Here's how the part is built. I have some questions about the finished solid (model axes, mm). Face numbers are marked on the shaded views. A direction names the side the tool comes from. Coordinates: 2 decimals unless noted, no trailing zeros. Write each loop counter-clockwise with the first axis right and the second up, starting at its lowest first coordinate (ties: lowest second). Pieces come first, ordered by that corner, then holes.
Item 1: If I drill on line 1 (X direction, y = -5, z = 4.5); line 2 (X direction, y = -3.75, z = 4); line 3 (X direction, y = -25.5, z = 5.5), over which ranges is the centre line in solid material (lowest first)?
Item 2: If we section it at B-B (z = -21.5): Please give me the cut outline in (x, y) (3 decimals).
Item 3: We'd pull the mould along Z, two halves only. Please class the marked faces 1, 2 and 3: +Z half, -Z half, draft (parallel to the pull), parting line (faces both ways), or undercut.
Item 4: If we section it at A-A (y = -13): Please give me the cut outline in (x, z), then the cut area to 3 significant figures.
Item 5: If we section it at D-D (y = -23): Please give me the cut outline in (x, z), then the cut area to 3 significant figures.
Item 6: For the marked faces 4, 5 and 6, which set-ups out of +Z, -Z, +X, -X, +Y, -Y let a thin tool reach every point of the face, with its end or its side?
Item 7: I'm going to push flat-ended pins straight in: pin 1 Ø18 at (x, z) = (-15, 0) entering from -Y; pin 2 Ø6 at (x, y) = (-22.5, -24) entering from -Z; pin 3 Ø3 at (x, y) = (-25, -8.5) entering from -Z. Where does each tip first touch, or does it pass through?
Item 8: If we section it at C-C (x = -16): Please give me the cut outline in (y, z), then the cut area to 3 significant figures.
from build123d import *

# Parameters (mm, degrees)
F1_DEPTH = 1
F2_DEPTH = 20
F3_DEPTH = 27


with BuildPart() as f1:
    # F0 (on Front) → F1 (new body)
    with BuildSketch(Plane.XZ):
        with BuildLine():
            ThreePointArc((28.6, -10.2), (24.1268833673, 14.3422452914), (0, 8))
            ThreePointArc((0, 8), (-24.1268833673, 14.3422452914), (-28.6, -10.2))
            Line((-28.6, -10.2), (0, -48.3333333333))
            Line((0, -48.3333333333), (28.6, -10.2))
        make_face()
        with BuildLine():
            ThreePointArc((-27.64, -9.48), (-22.3177005427, 14.0032588624), (0, 4.9638694584))
            ThreePointArc((0, 4.9638694584), (22.3177005427, 14.0032588624), (27.64, -9.48))
            Line((27.64, -9.48), (0, -46.3333333333))
            Line((0, -46.3333333333), (-27.64, -9.48))
        make_face(mode=Mode.SUBTRACT)
        with BuildLine():
            ThreePointArc((27.64, -9.48), (22.3177005427, 14.0032588624), (0, 4.9638694584))
            ThreePointArc((0, 4.9638694584), (-22.3177005427, 14.0032588624), (-27.64, -9.48))
            Line((-27.64, -9.48), (0, -46.3333333333))
            Line((0, -46.3333333333), (27.64, -9.48))
        make_face()
        with BuildLine():
            ThreePointArc((-27, -9), (-19.7434164903, 14.2302494708), (0, 0))
            ThreePointArc((0, 0), (19.7434164903, 14.2302494708), (27, -9))
            Line((27, -9), (0, -45))
            Line((0, -45), (-27, -9))
        make_face(mode=Mode.SUBTRACT)
        with BuildLine():
            ThreePointArc((27, -9), (19.7434164903, 14.2302494708), (0, 0))
            ThreePointArc((0, 0), (-19.7434164903, 14.2302494708), (-27, -9))
            Line((-27, -9), (0, -45))
            Line((0, -45), (27, -9))
        make_face()
    extrude(amount=F1_DEPTH)

    # F0 (on Front) → F2 (join)
    with BuildSketch(Plane.XZ):
        with BuildLine():
            ThreePointArc((28.6, -10.2), (24.1268833673, 14.3422452914), (0, 8))
            ThreePointArc((0, 8), (-24.1268833673, 14.3422452914), (-28.6, -10.2))
            Line((-28.6, -10.2), (0, -48.3333333333))
            Line((0, -48.3333333333), (28.6, -10.2))
        make_face()
        with BuildLine():
            ThreePointArc((-27.64, -9.48), (-22.3177005427, 14.0032588624), (0, 4.9638694584))
            ThreePointArc((0, 4.9638694584), (22.3177005427, 14.0032588624), (27.64, -9.48))
            Line((27.64, -9.48), (0, -46.3333333333))
            Line((0, -46.3333333333), (-27.64, -9.48))
        make_face(mode=Mode.SUBTRACT)
    extrude(amount=F2_DEPTH)

    # F0 (on Front) → F3 (join)
    with BuildSketch(Plane.XZ):
        with BuildLine():
            ThreePointArc((27.64, -9.48), (22.3177005427, 14.0032588624), (0, 4.9638694584))
            ThreePointArc((0, 4.9638694584), (-22.3177005427, 14.0032588624), (-27.64, -9.48))
            Line((-27.64, -9.48), (0, -46.3333333333))
            Line((0, -46.3333333333), (27.64, -9.48))
        make_face()
        with BuildLine():
            ThreePointArc((-27, -9), (-19.7434164903, 14.2302494708), (0, 0))
            ThreePointArc((0, 0), (19.7434164903, 14.2302494708), (27, -9))
            Line((27, -9), (0, -45))
            Line((0, -45), (-27, -9))
        make_face(mode=Mode.SUBTRACT)
    extrude(amount=F3_DEPTH)


solid = f1.part
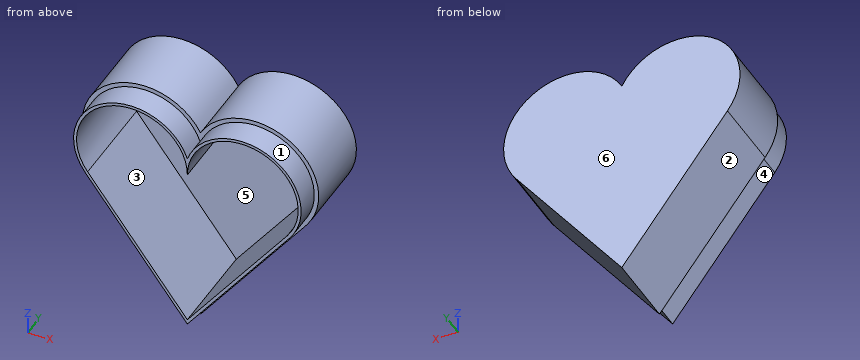
Answer list:
1. line 1: x = -31.39 to -29.31, -0.69 to 0.69, 29.31 to 31.39
1. line 2: x = -31.52 to -29.46, -0.54 to 0.54, 29.46 to 31.52
1. line 3: x = -29.81 to -28.96, -1.04 to -0.19, 0.19 to 1.04, 28.96 to 29.81
2. outline: (-20.125, -20) - (-18.625, -20) - (-18.625, -27) - (-17.625, -27) - (-17.625, -1) - (17.625, -1) - (17.625, -27) - (18.625, -27) - (18.625, -20) - (20.125, -20) - (20.125, 0) - (-20.125, 0) - close
3. face 1: parting line
3. face 2: -Z half
3. face 3: undercut
4. outline: (-28.6, -10.2) - (0, -48.33) - (28.6, -10.2) arc R17 ccw (long way) to (0, 8) arc R17 ccw (long way) to start; hole (-27, -9) - (0, -45) - (27, -9) arc R15 ccw (long way) to (0, 0) arc R15 ccw (long way) to start
4. area: 406 mm2
5. outline: (-27.64, -9.48) - (0, -46.33) - (27.64, -9.48) arc R15.8 ccw (long way) to (0, 4.96) arc R15.8 ccw (long way) to start; hole (-27, -9) - (0, -45) - (27, -9) arc R15 ccw (long way) to (0, 0) arc R15 ccw (long way) to start
5. area: 161 mm2
6. face 4: -Z, -X, -Y
6. face 5: -Y
6. face 6: +Z, -Z, +X, -X, +Y
7. pin 1: stops at y = -1
7. pin 2: stops at z = -20.33
7. pin 3: stops at z = -17
8. outline: (-27, -25) - (-20, -25) - (-20, -27) - (0, -27) - (0, 16.97) - (-20, 16.97) - (-20, 15.77) - (-27, 15.77) - (-27, 14.97) - (-1, 14.97) - (-1, -23.67) - (-27, -23.67) - close
8. area: 160 mm2
